```python
from build123d import *

# Parameters (mm, degrees)
SCHIZZO1_W                   = 121
SCHIZZO1_H                   = 48.8
ESTRUSIONE_ESTRUSIONE1_DEPTH = 2
TAGLIO_ESTRUSIONE1_DEPTH     = 12


with BuildPart() as part:
    # Schizzo1 → Estrusione-Estrusione1 (new body)
    with BuildSketch(Plane.XY):
        with Locations((60.5, 24.4)):
            Rectangle(SCHIZZO1_W, SCHIZZO1_H)
    extrude(amount=ESTRUSIONE_ESTRUSIONE1_DEPTH)

    # Schizzo2 → Taglio-Estrusione1 (cut)
    with BuildSketch(Plane.XY.offset(2)):
        with BuildLine():
            Line((126.922454277, 4.622930456), (115.077545723, 4.622930456))
            ThreePointArc((115.077545723, 4.622930456), (111.052124488, 8.64835169), (115.077545723, 12.673772925))
            Line((115.077545723, 12.673772925), (126.922454277, 12.673772925))
            ThreePointArc((126.922454277, 12.673772925), (130.947875512, 8.64835169), (126.922454277, 4.622930456))
        make_face()
    extrude(amount=-TAGLIO_ESTRUSIONE1_DEPTH, mode=Mode.SUBTRACT)


solid = part.part
```
Check sheet for the modelled part. Datum: model origin and axes. Units: mm. A direction names the side the tool comes from. Round coordinates to 2 decimals unless told otherwise and drop trailing zeros. Loops run counter-clockwise (first coordinate to the right, second up) from the corner with the lowest first, then second, coordinate; pieces in that order, holes last. Notation, with made-up numbers: (28, 20) -> (73, 20) arc R16 cw to (73, 40) -> close; hole circle Ø4 at (16, 47). An arc over 180 degrees is marked (long way). Answer in a Markdown table with one row per item.
Q1. Release check for a two-part mould opening along Y. For faces 1 (the face through (121, 30, 1)), 2 (the face through (60, 48.8, 1)), 3 (the face through (60, 0, 1)), 4 (the face through (118, 4.623, 1)) record: released by +Y, released by -Y, zero draft, split by the parting line, or undercut.
Data:
| item | result |
|---|---|
| face 1 | zero draft |
| face 2 | released by +Y |
| face 3 | released by -Y |
| face 4 | undercut |
Q2. Thickness scan on L1, parallel to X at y = 8.5, z = 0.85; L2, parallel to Y at x = 111.5, z = 0.6. Record the ranges inside material, lowest first.
Data:
| item | result |
|---|---|
| L1 | x = 0 to 111.05 |
| L2 | y = 0 to 6.8, 10.49 to 48.8 |
Q3. Sectioned sample at A-A on y = 6. Enter the section's corners in (x, z).
Data:
| item | result |
|---|---|
| outline | (0, 0) -> (112.05, 0) -> (112.05, 2) -> (0, 2) -> close |
Q4. Go/stop test with a flat-tipped pin: P1, Ø5, axis at x = 73.5, y = 37, coming from the -Z side. Record where the tip stops, or that it passes through.
Data:
| item | result |
|---|---|
| P1 | stops at z = 0 |
Q5. Set-up check for faces 5 (the face through (118, 12.674, 1)), 6 (the face through (60, 25, 0)): record each of +Z, -Z, +X, -X, +Y, -Y from which the full face is reachable in a straight line by a thin tool's end or side.
Data:
| item | result |
|---|---|
| face 5 | +Z, -Z, +X |
| face 6 | -Z, +X, -X, +Y, -Y |
